Source: CAD feature listing. Evaluate the final solid. Frame: model axes, mm. Give positions to 0.01 mm unless a question says otherwise; leave off trailing zeros. Order: outer loops, then holes, each group sorted by start corner. A loop starts at its lowest first (then second) coordinate and runs counter-clockwise, first axis right, second up.
from build123d import *

# Parameters (mm, degrees)
BOSS_EXTRUDE1_DEPTH     = 6.35
SKETCH3_W               = 107.95
SKETCH3_H               = 76.2
BOSS_EXTRUDE2_DEPTH     = 6.35
FILLET1_R               = 5.08
CUT_EXTRUDE1_REACH      = 199.668
SKETCH4_R               = 14.2875
F_1_4_CLEARANCE_HOLE1_D = 6.7564
SKETCH12_R              = 4.2164
CUT_EXTRUDE2_DEPTH      = 6.35


with BuildPart() as part:
    # Sketch2 → Boss-Extrude1 (new body)
    with BuildSketch(Plane.XY):
        with BuildLine():
            Line((50.8, 63.5), (-139.7, 63.5))
            Line((-139.7, 63.5), (-139.7, 24.9428))
            ThreePointArc((-139.7, 24.9428), (-132.170466199, 1.196645543), (-112.333373337, -13.871980059))
            Line((-112.333373337, -13.871980059), (-17.064303956, -47.848192552))
            ThreePointArc((-17.064303956, -47.848192552), (29.272626795, -41.518108344), (50.8, 0))
            Line((50.8, 0), (50.8, 63.5))
        make_face()
    extrude(amount=-BOSS_EXTRUDE1_DEPTH)

    # Sketch3 → Boss-Extrude2 (add)
    with BuildSketch(Plane.XY):
        with Locations((-85.725, 101.6)):
            Rectangle(SKETCH3_W, SKETCH3_H)
    extrude(amount=-BOSS_EXTRUDE2_DEPTH)

    # Fillet1
    fillet1_edges = [part.edges().sort_by_distance(p)[0] for p in [
        (50.8, 63.5, -3.175),
        (-31.75, 139.7, -3.175),
        (-139.7, 139.7, -3.175),
        (-31.75, 63.5, -3.175),
    ]]
    fillet(fillet1_edges, radius=FILLET1_R)

    # Sketch4 → Cut-Extrude1 (cut, up to next)
    with BuildSketch(Plane.XY, mode=Mode.PRIVATE) as cut_extrude1_sk1:
        Circle(SKETCH4_R)
    cut_extrude1_tool1 = extrude(cut_extrude1_sk1.sketch, amount=-CUT_EXTRUDE1_REACH, mode=Mode.PRIVATE) & part.part
    add(cut_extrude1_tool1.solids().sort_by_distance((0, 0, 0))[0], mode=Mode.SUBTRACT)

    # 1/4 Clearance Hole1 (through all)
    with Locations(Plane.XY):
        with Locations((-33.671992271, -35.183583732), (-92.344956452, -14.258795534), (-130.175, 53.975), (-15.875, 53.975), (41.275, 53.975)):
            Hole(F_1_4_CLEARANCE_HOLE1_D / 2)

    # Sketch12 → Cut-Extrude2 (cut)
    with BuildSketch(Plane.XY):
        with Locations((-123.825, 120.65)):
            Circle(SKETCH12_R)
        with Locations((-123.825, 82.55)):
            Circle(SKETCH12_R)
        with Locations((-85.725, 120.65)):
            Circle(SKETCH12_R)
        with Locations((-85.725, 82.55)):
            Circle(SKETCH12_R)
        with Locations((-47.625, 82.55)):
            Circle(SKETCH12_R)
        with Locations((-47.625, 120.65)):
            Circle(SKETCH12_R)
    extrude(amount=-CUT_EXTRUDE2_DEPTH, mode=Mode.SUBTRACT)


solid = part.part
(1) Section C-C, the plane z = -4.25. Count the separate pieces of the cut face and the enclosed holes in it, plus the area to 3 significant figures.
(2) Section D-D, the plane y = 72.5. Return loops of the section in (x, z), plus the area to 3 significant figures.
(3) Line query: line 1 along X through (y, z) = (55, -3); line 2 along Y through (x, z) = (-124, -3.5); line 3 along X through (y, z) = (122.5, -2). Output: solid intervals per line, ascending.
(4) Section B-B, the plane x = 0. Return loops of the section in (y, z).
(5) Pin query (flat end, axial travel): pin 1 Ø5.5 at (x, y) = (41.275, 53.975) entering from -Z; pin 2 Ø3 at (y, z) = (115, -4.5) entering from +X; pin 3 Ø9.5 at (x, y) = (-123.825, 120.65) entering from -Z; pin 4 Ø1.9 at (x, z) = (-5.5, -2.5) entering from +Y. Return the tip coordinate at first contact, or that it passes through.
(6) Draft query along Y for faces 1 (the cylindrical face through (-86.639, 78.434, -3.131)), 2 (the cylindrical face through (-132.373, 1.487, -3.131)), 3 (the cylindrical face through (-138.251, 138.172, -3.219)). Return one class per face: +Y half, -Y half, draft (parallel to the pull), parting line (faces both ways), or undercut.
(7) Section A-A, the plane y = 120.65. Return loops of the section in (x, z), plus the area to 3 significant figures.
Checks:
1. separate pieces: 1
1. enclosed holes: 12
1. area: 25,100 mm2
2. outline: (-139.7, -6.35) - (-31.75, -6.35) - (-31.75, 0) - (-139.7, 0) - close
2. area: 685 mm2
3. line 1: x = -139.7 to -133.39, -126.96 to -19.09, -12.66 to 38.06, 44.49 to 50.8
3. line 2: y = -7.42 to 78.34, 86.76 to 116.44, 124.86 to 139.7
3. line 3: x = -139.7 to -127.61, -120.04 to -89.51, -81.94 to -51.41, -43.84 to -31.75
4. outline: (-50.8, -6.35) - (-14.29, -6.35) - (-14.29, 0) - (-50.8, 0) - close; (14.29, -6.35) - (63.5, -6.35) - (63.5, 0) - (14.29, 0) - close
5. pin 1: passes through
5. pin 2: stops at x = -31.75
5. pin 3: stops at z = -6.35
5. pin 4: stops at y = 63.5
6. face 1: undercut
6. face 2: -Y half
6. face 3: +Y half
7. outline: (-139.7, -6.35) - (-128.04, -6.35) - (-128.04, 0) - (-139.7, 0) - close; (-119.61, -6.35) - (-89.94, -6.35) - (-89.94, 0) - (-119.61, 0) - close; (-81.51, -6.35) - (-51.84, -6.35) - (-51.84, 0) - (-81.51, 0) - close; (-43.41, -6.35) - (-31.75, -6.35) - (-31.75, 0) - (-43.41, 0) - close
7. area: 525 mm2
